The listing builds one solid part. Answer for the finished solid, in the listing's coordinates (mm). Face numbers are marked on the shaded views. Give positions to 0.01 mm unless a question says otherwise; leave off trailing zeros. Write each loop counter-clockwise with the first axis right and the second up, starting at its lowest first coordinate (ties: lowest second). Pieces come first, ordered by that corner, then holes. Notation, with made-up numbers: (5.5, 0.25) - (48.5, 0.25) arc R36 ccw to (48.5, 38.25) - close; hole circle Ø4 at (-33.5, 70). An arc over 180 degrees is marked (long way). One line per question, with ' | ' between items. Start each with the question number.
1. A cutting plane is placed at B-B (z = 16.5). Determine the outline of the cut face in (x, y).
2. A cutting plane is placed at A-A (z = 19.5). Determine the outline of the cut face in (x, y).
3. Given P1, Ø1.5, axis at x = 2, z = 12, coming from the -Y side; P2, Ø1, axis at y = 1.5, z = 23.5, coming from the -X side; P3, Ø1.5, axis at y = 3, z = 17, coming from the +X side, each flat-ended and moving along its own axis, determine where each tip first touches the part or whether it passes through.
4. The mould has two halves that part along Z. Classify the marked faces 1 and 2: +Z half, -Z half, draft (parallel to the pull), parting line (faces both ways), or undercut.
5. Find the intervals of material crossed by L1, parallel to Z at x = -3.25, y = 3; L2, parallel to Z at x = -2.75, y = -3; L3, parallel to Y at x = -4, z = 9.5, in increasing order. Write a range as from..to.
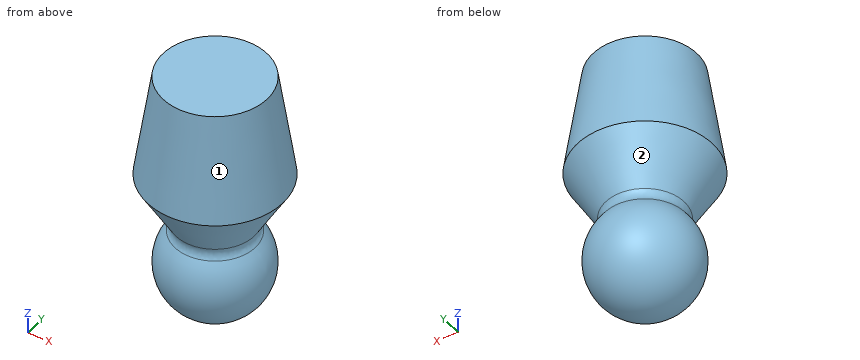
```python
from build123d import *

# Parameters (mm, degrees)
FILLET005_R = 1


with BuildPart() as cone001:
    # Cone001 → Cone001 (revolve)
    with BuildSketch(Plane(origin=(0, 0, 17), x_dir=(1, 0, 0), z_dir=(0, -1, 0))):
        Polygon((0, 0), (6.5, 0), (5, 10), (0, 10), align=None)
    revolve(axis=Axis((0, 0, 17), (0, 0, 1)))


with BuildPart() as cone:
    # Cone → Cone (revolve)
    with BuildSketch(Plane(origin=(0, 0, 11), x_dir=(1, 0, 0), z_dir=(0, -1, 0))):
        Polygon((0, 0), (3, 0), (6.5, 6), (0, 6), align=None)
    revolve(axis=Axis((0, 0, 11), (0, 0, 1)))


with BuildPart() as shaft_in_place:
    # Sphere → Sphere (revolve)
    with BuildSketch(Plane(origin=(0, 0, 8), x_dir=(1, 0, 0), z_dir=(0, -1, 0))):
        with BuildLine():
            ThreePointArc((0, -5), (5, 0), (0, 5))
            Line((0, 5), (0, -5))
        make_face()
    revolve(axis=Axis((0, 0, 8), (0, 0, 1)))

    # Fusion: union Cone001, Cone
    add(cone001.part)
    add(cone.part)


with BuildPart() as shaft_in_place_1:
    # Fusion placement: moved
    add(shaft_in_place.part.moved(Location((0, 0, 0.5))))

    # Fillet005
    fillet005_edges = [shaft_in_place_1.edges().sort_by_distance(p)[0] for p in [
        (-3.392555, 0, 12.172951),
    ]]
    fillet(fillet005_edges, radius=FILLET005_R)


solid = shaft_in_place_1.part
```
Determined:
1) outline: circle Ø11.83 at (0, 0)
2) outline: circle Ø12.4 at (0, 0)
3) P1: y = -3.77 | P2: x = -5.54 | P3: x = 6.02
4) face 1: +Z half | face 2: undercut
5) L1: 6.17..10.83, 13.94..27.5 | L2: 5.6..11.4, 13.33..27.5 | L3: -2.83..2.83
